Work out the finished part from the listing and answer in its coordinate system (mm). A direction names the side the tool comes from. Coordinates: 2 decimals unless noted, no trailing zeros. Loops run counter-clockwise (first coordinate to the right, second up) from the corner with the lowest first, then second, coordinate; pieces in that order, holes last. Notation, with made-up numbers: M 49.5,-37.5 L 94.5,-37.5 A33 cw 94.5,1.5 Z; hole C 66,71.25 d6. An arc over 180 degrees is marked long. Write each question's results on one line, items separated by ' | '.
```python
from build123d import *

# Parameters (mm, degrees)
CROQUIS1_W              = 798
CROQUIS1_H              = 400
CROQUIS1_R              = 9
SALIENTE_EXTRUIR1_DEPTH = 50.8
VACIADO1_T              = -1.9
CROQUIS2_W              = 794.2
CROQUIS2_H              = 396.2
CORTAR_EXTRUIR1_DEPTH   = 48.9


with BuildPart() as part:
    # Croquis1 → Saliente-Extruir1 (new body)
    with BuildSketch(Plane.XY):
        with Locations((-399, 200)):
            Rectangle(CROQUIS1_W, CROQUIS1_H)
        with Locations((-599, 355)):
            Circle(CROQUIS1_R, mode=Mode.SUBTRACT)
        with Locations((-599, 246.5)):
            Circle(CROQUIS1_R, mode=Mode.SUBTRACT)
        with Locations((-599, 104)):
            Circle(CROQUIS1_R, mode=Mode.SUBTRACT)
        with Locations((-199, 104)):
            Circle(CROQUIS1_R, mode=Mode.SUBTRACT)
        with Locations((-199, 355)):
            Circle(CROQUIS1_R, mode=Mode.SUBTRACT)
    extrude(amount=SALIENTE_EXTRUIR1_DEPTH)

    # Vaciado1
    vaciado1_openings = [part.faces().sort_by_distance(p)[0] for p in [
        (-398.839920182, 199.86833435, 50.8),
    ]]
    offset(amount=VACIADO1_T, openings=vaciado1_openings, kind=Kind.INTERSECTION)

    # Croquis2 → Cortar-Extruir1 (cut)
    with BuildSketch(Plane.XY.offset(50.8)):
        with Locations((-399, 200)):
            Rectangle(CROQUIS2_W, CROQUIS2_H)
    extrude(amount=-CORTAR_EXTRUIR1_DEPTH, mode=Mode.SUBTRACT)


solid = part.part
```
1) Find section A-A, the plane x = -199. Give the vertices of the cut face in (y, z), and give its area (3 significant figures).
Check result:
outline: M 0,0 L 95,0 L 95,1.9 L 1.9,1.9 L 1.9,50.8 L 0,50.8 Z; M 113,0 L 346,0 L 346,1.9 L 113,1.9 Z; M 364,0 L 400,0 L 400,50.8 L 398.1,50.8 L 398.1,1.9 L 364,1.9 Z | area: 877 mm^2
2) Find section B-B, the plane x = -599. Give the vertices of the cut face in (y, z).
Check result:
outline: M 0,0 L 95,0 L 95,1.9 L 1.9,1.9 L 1.9,50.8 L 0,50.8 Z; M 113,0 L 237.5,0 L 237.5,1.9 L 113,1.9 Z; M 255.5,0 L 346,0 L 346,1.9 L 255.5,1.9 Z; M 364,0 L 400,0 L 400,50.8 L 398.1,50.8 L 398.1,1.9 L 364,1.9 Z
3) Find section C-C, the plane y = 104. Give the vertices of the cut face in (x, z).
Check result:
outline: M -798,0 L -608,0 L -608,1.9 L -796.1,1.9 L -796.1,50.8 L -798,50.8 Z; M -590,0 L -208,0 L -208,1.9 L -590,1.9 Z; M -190,0 L 0,0 L 0,50.8 L -1.9,50.8 L -1.9,1.9 L -190,1.9 Z
4) For a pull along Y with two mould halves and no side action, classify faces 1 (the face through (-405, 0, 25)), 2 (the face through (-405, 400, 25)), 3 (the face through (-590.686, 243.053, 0.937)), 4 (the face through (-405, 203, 0)) as released by +Y, released by -Y, zero draft, split by the parting line, or undercut.
Check result:
face 1: released by -Y | face 2: released by +Y | face 3: undercut | face 4: zero draft
5) Find section D-D, the plane y = 246.5. Give the vertices of the cut face in (x, z), and give its area (3 significant figures).
Check result:
outline: M -798,0 L -608,0 L -608,1.9 L -796.1,1.9 L -796.1,50.8 L -798,50.8 Z; M -590,0 L 0,0 L 0,50.8 L -1.9,50.8 L -1.9,1.9 L -590,1.9 Z | area: 1,670 mm^2
6) Straight lines are drawn through the part: probe 1 along Y at (x, z) = (-199, 0.65); probe 2 along X at (y, z) = (355, 0.5); probe 3 along Y at (x, z) = (-599, 0.8). For each, find the intervals that lie inside material, in ascending order. Write a range as [from, to].
Check result:
probe 1: [0, 95], [113, 346], [364, 400] | probe 2: [-798, -608], [-590, -208], [-190, 0] | probe 3: [0, 95], [113, 237.5], [255.5, 346], [364, 400]
7) Which of the six approach directions +Z, -Z, +X, -X, +Y, -Y give full straight-line access (tool end or side, diameter ignored) to faces 5 (the face through (-798, 197, 25)), 6 (the face through (-405, 1.9, 26))?
Check result:
face 5: +Z, -Z, -X, +Y, -Y | face 6: +Z
8) Given pin 1 Ø12 at (x, y) = (-369.5, 228.5) entering from +Z, flat-ended and moving along its own axis, determine where the tip first touches the part or whether it passes through.
Check result:
pin 1: z = 1.9
